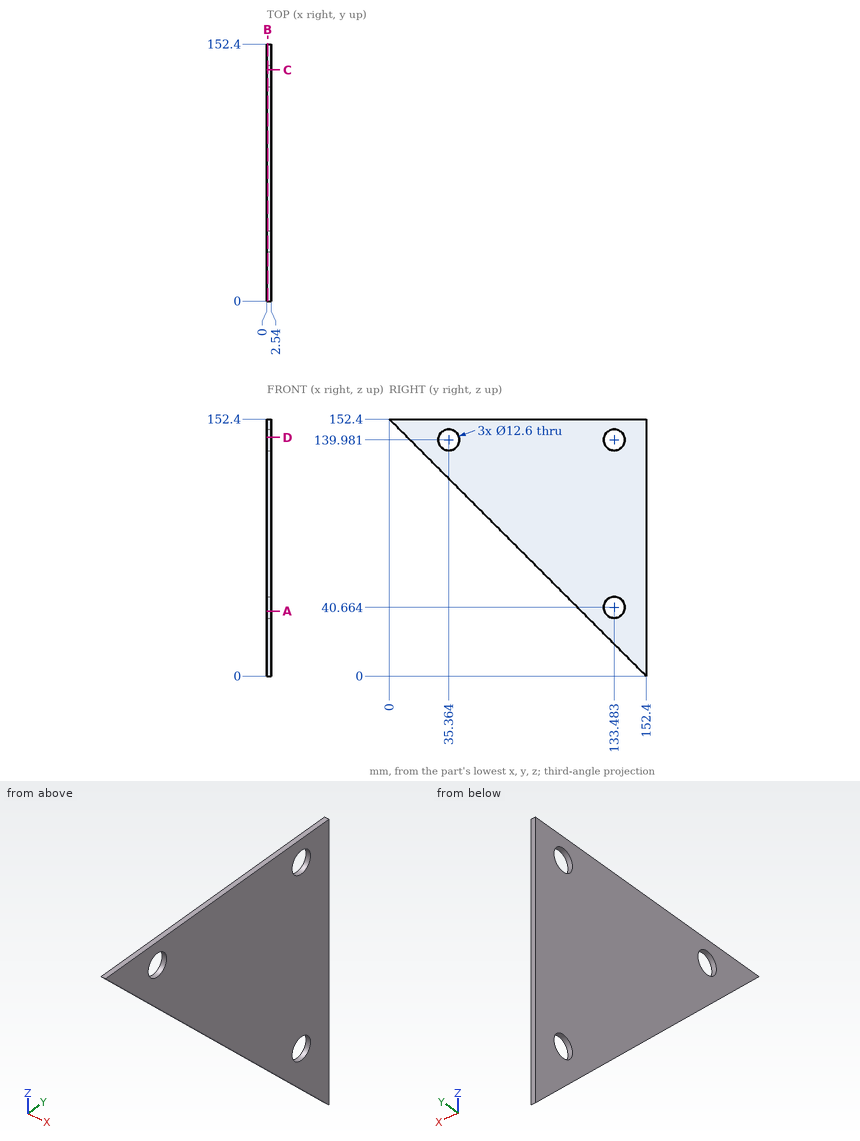
Geometry: see drawing. Coordinates: mm, zero at the bounding-box minimum. Coordinates: 2 decimals unless noted, no trailing zeros. Loops run counter-clockwise (first coordinate to the right, second up) from the corner with the lowest first, then second, coordinate; pieces in that order, holes last. Notation, with made-up numbers: M -16.75,55 L 14.25,55 A22 cw 14.25,82 Z; hole C 8.5,20 d3. An arc over 180 degrees is marked long. Put each result on its own line as item: value. Start each with the question number.
1) Ray query, L1, parallel to Y at x = 1.15, z = 145 (1 decimal); L2, parallel to Z at x = 2.4, y = 138 (1 decimal); L3, parallel to Z at x = 1.45, y = 31 (1 decimal). Return the intervals inside material, ascending. Write a range as from..to.
2) Cut plane C-C on y = 137. Return the cut outline in (x, z).
3) Cut plane A-A on z = 38.5. Return the cut outline in (x, y).
4) Cut plane B-B on x = 0.4. Return the cut outline in (y, z) (1 decimal), then the cut area to 3 significant figures.
5) Contact query for flat-ended pins moving along their axis: pin 1 Ø16.5 at (y, z) = (133.48, 40.66) entering from -X; pin 2 Ø1.5 at (x, z) = (1.5, 129) entering from -Y. Output: stop coordinate, or through.
6) Cut plane D-D on z = 141.5. Return the cut outline in (x, y).
The answers:
1. L1: y = 7.4..31.6, 39.2..129.7, 137.3..152.4
1. L2: z = 14.4..36.3, 45.1..135.6, 144.4..152.4
1. L3: z = 121.4..135.4, 144.5..152.4
2. outline: M 0,15.4 L 2.54,15.4 L 2.54,35.44 L 0,35.44 Z; M 0,45.89 L 2.54,45.89 L 2.54,134.75 L 0,134.75 Z; M 0,145.21 L 2.54,145.21 L 2.54,152.4 L 0,152.4 Z
3. outline: M 0,113.9 L 2.54,113.9 L 2.54,127.57 L 0,127.57 Z; M 0,139.4 L 2.54,139.4 L 2.54,152.4 L 0,152.4 Z
4. outline: M 0,152.4 L 152.4,0 L 152.4,152.4 Z; hole C 35.4,140 d12.6; hole C 133.5,40.7 d12.6; hole C 133.5,140 d12.6
4. area: 11,200 mm²
5. pin 1: stops at x = 0
5. pin 2: stops at y = 22.65
6. outline: M 0,10.9 L 2.54,10.9 L 2.54,29.25 L 0,29.25 Z; M 0,41.48 L 2.54,41.48 L 2.54,127.37 L 0,127.37 Z; M 0,139.6 L 2.54,139.6 L 2.54,152.4 L 0,152.4 Z
